The model under review builds one solid part; all positions refer to its coordinate system, in mm. A direction names the side the tool comes from. Round coordinates to 2 decimals unless told otherwise and drop trailing zeros. Write each loop counter-clockwise with the first axis right and the second up, starting at its lowest first coordinate (ties: lowest second). Pieces come first, ordered by that corner, then holes. Notation, with made-up numbers: (65.5, -2) -> (76.5, -2) arc R22 ccw to (76.5, 22) -> close; hole circle Ø3 at (-30.5, 64.25). An arc over 180 degrees is marked (long way). Return JSON: item names as keys, results as strings. Group by question number.
1. Take a section at B-B, the plane x = 3. Write out the cut boundary in (y, z).
2. Clearance check with flat-ended pins moving along their axes: P1, Ø1.6, axis at x = 22, z = -2.5, coming from the +Y side; P2, Ø2, axis at x = 14.5, y = 3.5, coming from the +Z side; P3, Ø3, axis at y = 2, z = -12, coming from the +X side; P4, Ø2.5, axis at y = 4, z = -19, coming from the -X side. State where each tip first meets the part, or that it passes through.
3. For line 1 along Z through (x, y) = (22.25, 1.5); line 2 along Z through (x, y) = (22, 5.75); line 3 along Z through (x, y) = (3, 3.25), list the stretches that pass through material, from the lowest coordinate up. Write a range as from..to.
4. Mouldability with a two-part tool opening along Z and no side actions: class faces 1 (the cylindrical face through (21, 4.2, -2.5)), 2 (the flat face through (15, 4, -18)), 3 (the flat face through (12, 3, -5)) as pulls with the +Z half, pulls with the -Z half, needs draft (parallel to the pull), parting line crosses it, or undercut.
5. Tool access review of faces 4 (the flat face through (8, 4, -10)), 5 (the cylindrical face through (22.5, 6.5, -12.6)), 6 (the cylindrical face through (2.2, 4.2, -3.1)), 7 (the cylindrical face through (12.6, 6.5, -2.5)): name each direction out of +Z, -Z, +X, -X, +Y, -Y from which nothing blocks a thin tool from reaching the whole face with its end or side.
6. Take a section at A-A, the plane z = -2.5. Write out the cut boundary in (x, y), then the cut area to 3 significant figures.
7. Take a section at D-D, the plane y = 5.75. Write out the cut boundary in (x, z), then the cut area to 3 significant figures.
8. Take a section at C-C, the plane z = -22. Write out the cut boundary in (x, y).
Autodesk Fusion 360 part; units mm, degrees
sketch "Sketch1" plane through (0, 0, 0) normal (0, 1, 0) x (1, 0, 0)
  line L0 (0, 0) -> (25, 0)
  line L1 (25, 0) -> (25, 25)
  line L2 (25, 25) -> (15, 25)
  line L3 (0, 10) -> (0, 0)
  line L4 (15, 25) -> (15, 10)
  line L5 (15, 10) -> (0, 10)
  dimension "d13" = 25
  dimension "d14" = 25
  dimension "d15" = 15
extrude "Extrude1" add sketch "Sketch1" along normal blind 8.5
sketch "Sketch2" plane through (25, 0, 0) normal (1, 0, 0) x (0, 0, -1)
  line L0 (0, 0) -> (25, 0)
  line L1 (25, 0) -> (25, 8.5)
  line L2 (25, 8.5) -> (0, 8.5)
  line L3 (0, 8.5) -> (0, 0)
  arc A0 (19, 0) -> (6, 0) centre (12.5, 0) ccw
  line L4 (6, 0) -> (19, 0)
  dimension "d5" = 13
extrude "Extrude2" cut sketch "Sketch2" against normal blind 5 contours L0 A0 L4
sketch "Sketch3" plane through (0, 0, 0) normal (0, 0, 1) x (1, 0, 0)
  line L0 (0, 0) -> (25, 0)
  line L1 (25, 0) -> (25, 8.5)
  line L2 (25, 8.5) -> (0, 8.5)
  line L3 (0, 8.5) -> (0, 0)
  arc A0 (19, 0) -> (6, 0) centre (12.5, 0) ccw
  line L4 (6, 0) -> (19, 0)
  dimension "d8" = 13
extrude "Extrude3" cut sketch "Sketch3" against normal blind 5 contours L0 A0 L4
sketch "Sketch4" plane through (0, 0, 0) normal (0, -1, 0) x (1, 0, 0)
  line L0 (19, 0) -> (19, -5)
  line L1 (19, -5) -> (6, -5)
  line L2 (6, -5) -> (6, 0)
  line L3 (6, 0) -> (0, 0)
  line L4 (0, 0) -> (0, -10)
  line L5 (0, -10) -> (15, -10)
  line L6 (15, -10) -> (15, -25)
  line L7 (15, -25) -> (25, -25)
  line L8 (25, -25) -> (25, -19)
  line L9 (25, -19) -> (20, -19)
  line L10 (20, -19) -> (20, -6)
  line L11 (20, -6) -> (25, -6)
  line L12 (25, -6) -> (25, 0)
  line L13 (25, 0) -> (19, 0)
  circle A0 centre (3, -2.5) radius 1
  line L14 (0, -2.5) -> (25, -2.5) construction
  line L15 (22, 0) -> (22, -25) construction
  line L16 (25, -22) -> (24.6457, -22)
  line L17 (24.6457, -22) -> (15, -22) construction
  line L18 (3, 0) -> (3, -10) construction
  circle A1 centre (22, -22) radius 1
  circle A2 centre (22, -2.5) radius 1
  dimension "d16" = 2
extrude "Extrude4" cut sketch "Sketch4" against normal through all contours A0 | A1 | A2
fillet "Fillet1" radius 0.2 2 edges at (0, 0, -5) (20, 0, -25)
Output:
{
 "1": {"outline": "(0, -10) -> (8.5, -10) -> (8.5, -3.5) -> (0, -3.5) -> close; (0, -1.5) -> (8.5, -1.5) -> (8.5, 0) -> (0, 0) -> close"},
 "2": {"P1": "passes through", "P2": "stops at z = -5", "P3": "stops at x = 20", "P4": "stops at x = 15"},
 "3": {"line 1": "z = -25..-22.97, -21.03..-18.82, -6.18..-3.47, -1.53..0", "line 2": "z = -25..-23, -21..-15.53, -9.47..-3.5, -1.5..0", "line 3": "z = -10..-3.5, -1.5..0"},
 "4": {"face 1": "undercut", "face 2": "needs draft", "face 3": "pulls with the +Z half"},
 "5": {"face 4": "-Z, -X, +Y, -Y", "face 5": "+X, -Y", "face 6": "+Y, -Y", "face 7": "+Z, -Y"},
 "6": {"outline": "(0, 0.2) arc R0.2 ccw to (0.2, 0) -> (2, 0) -> (2, 8.5) -> (0, 8.5) -> close; (4, 0) -> (6, 0) arc R6.5 cw to (19, 0) -> (21, 0) -> (21, 8.5) -> (4, 8.5) -> close; (23, 0) -> (25, 0) -> (25, 8.5) -> (23, 8.5) -> close", "area": "112 mm^2"},
 "7": {"outline": "(0, -10) -> (15, -10) -> (15, -25) -> (25, -25) -> (25, -15.53) -> (20, -15.53) -> (20, -9.47) -> (25, -9.47) -> (25, 0) -> (15.53, 0) -> (15.53, -5) -> (9.47, -5) -> (9.47, 0) -> (0, 0) -> close; hole circle Ø2 at (3, -2.5); hole circle Ø2 at (22, -22); hole circle Ø2 at (22, -2.5)", "area": "330 mm^2"},
 "8": {"outline": "(15, 0) -> (21, 0) -> (21, 8.5) -> (15, 8.5) -> close; (23, 0) -> (25, 0) -> (25, 8.5) -> (23, 8.5) -> close"}
}
